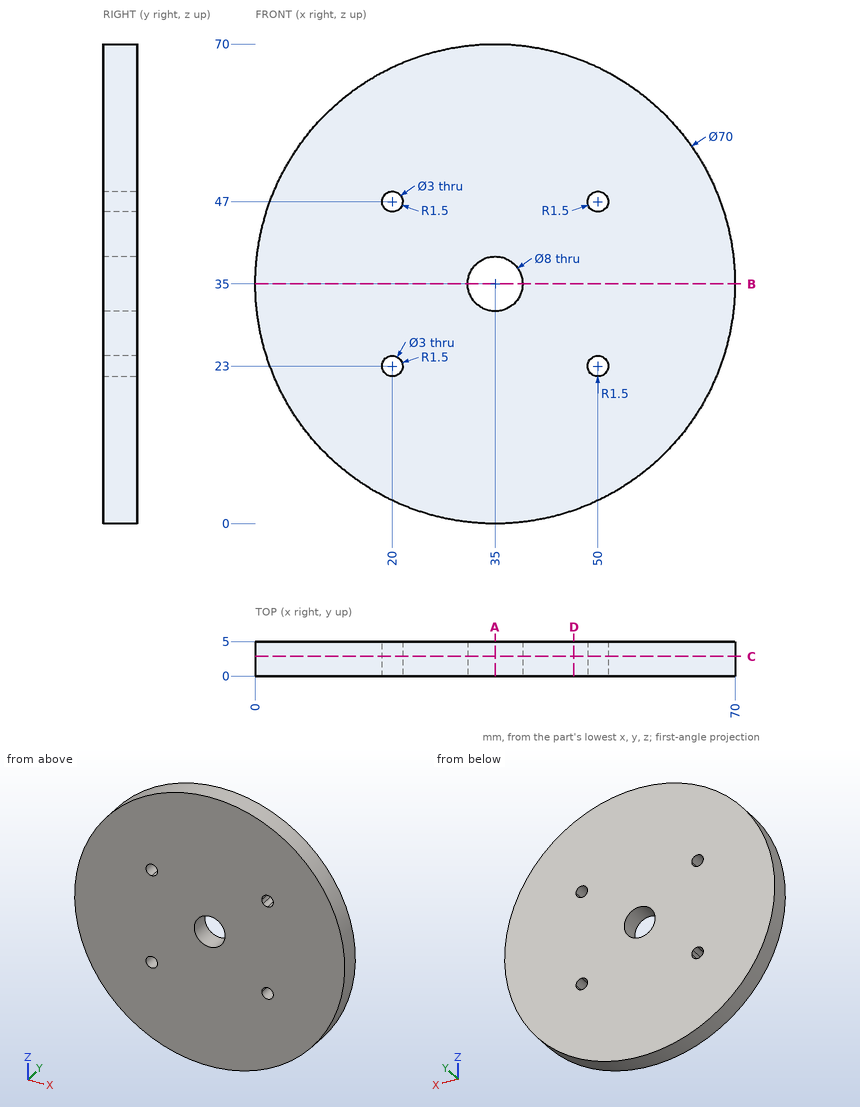
Check sheet for the drawn part. Datum: minimum x, y, z corner. Units: mm. Give positions to 0.01 mm unless a question says otherwise; leave off trailing zeros. Order: outer loops, then holes, each group sorted by start corner. A loop starts at its lowest first (then second) coordinate and runs counter-clockwise, first axis right, second up. Notation, with made-up numbers: (79.5, -15) -> (110.5, -15) arc R24 ccw to (110.5, 6) -> close; hole circle Ø1 at (59, 89). An arc over 180 degrees is marked (long way). Use a Markdown table: item, result.
1) Material ranges on probe 1 along X at (y, z) = (3.9, 47); probe 2 along Z at (x, y) = (20, 3.2); probe 3 along X at (y, z) = (1.5, 35), recorded low to high.
Results:
| item | result |
|---|---|
| probe 1 | 2.12 to 18.5, 21.5 to 48.5, 51.5 to 67.88 |
| probe 2 | 3.38 to 21.5, 24.5 to 45.5, 48.5 to 66.62 |
| probe 3 | 0 to 31, 39 to 70 |
2) Depth check by flat-ended pin: pin 1 Ø2 at (x, y) = (47.5, 4.5) entering from +Z; pin 2 Ø3 at (x, y) = (45.5, 2.5) entering from +Z; pin 3 Ø1.5 at (x, y) = (47, 4.5) entering from -Z. Enter the tip coordinate at first touch or a pass-through.
Results:
| item | result |
|---|---|
| pin 1 | z = 68.06 |
| pin 2 | z = 68.82 |
| pin 3 | z = 1.86 |
3) Section check C-C, the plane y = 2.85. Record the boundary of the cut face in (x, z).
Results:
| item | result |
|---|---|
| outline | circle Ø70 at (35, 35); hole circle Ø3 at (20, 23); hole circle Ø3 at (20, 47); hole circle Ø8 at (35, 35); hole circle Ø3 at (50, 23); hole circle Ø3 at (50, 47) |
4) Section check D-D, the plane x = 46.5. Record the boundary of the cut face in (y, z).
Results:
| item | result |
|---|---|
| outline | (0, 1.94) -> (5, 1.94) -> (5, 68.06) -> (0, 68.06) -> close |
5) Section check A-A, the plane x = 35. Record the boundary of the cut face in (y, z).
Results:
| item | result |
|---|---|
| outline | (0, 0) -> (5, 0) -> (5, 31) -> (0, 31) -> close; (0, 39) -> (5, 39) -> (5, 70) -> (0, 70) -> close |
6) Section check B-B, the plane z = 35. Record the boundary of the cut face in (x, y), then the cut area to 3 significant figures.
Results:
| item | result |
|---|---|
| outline | (0, 0) -> (31, 0) -> (31, 5) -> (0, 5) -> close; (39, 0) -> (70, 0) -> (70, 5) -> (39, 5) -> close |
| area | 310 mm² |
